Model file for the job. Use its own axes, mm. A direction names the side the tool comes from. Give positions to 0.01 mm unless a question says otherwise; leave off trailing zeros. Write each loop counter-clockwise with the first axis right and the second up, starting at its lowest first coordinate (ties: lowest second). Pieces come first, ordered by that corner, then holes.
```python
from build123d import *

# Parameters (mm, degrees)
SKETCH1_R           = 7.5
SKETCH1_R_2         = 1.7525
BOSS_EXTRUDE1_DEPTH = 6.35


with BuildPart() as part:
    # Sketch1 → Boss-Extrude1 (new body)
    with BuildSketch(Plane.XY):
        with BuildLine():
            Line((100, 110), (80, 110))
            Line((80, 110), (80, 78))
            Line((80, 78), (-3, 78))
            Line((-3, 78), (-3, 110))
            Line((-3, 110), (-27, 110))
            Line((-27, 110), (-27, 78))
            Line((-27, 78), (-110, 78))
            Line((-110, 78), (-110, 110))
            Line((-110, 110), (-130, 110))
            Line((-130, 110), (-130, 63.442887702))
            ThreePointArc((-130, 63.442887702), (-95, 0), (-130, -63.442887702))
            Line((-130, -63.442887702), (-130, -110))
            Line((-130, -110), (-110, -110))
            Line((-110, -110), (-110, -78))
            Line((-110, -78), (-27, -78))
            Line((-27, -78), (-27, -110))
            Line((-27, -110), (-3, -110))
            Line((-3, -110), (-3, -78))
            Line((-3, -78), (80, -78))
            Line((80, -78), (80, -110))
            Line((80, -110), (100, -110))
            Line((100, -110), (100, -63.442887702))
            ThreePointArc((100, -63.442887702), (65, 0), (100, 63.442887702))
            Line((100, 63.442887702), (100, 110))
        make_face()
        with Locations((32.5, 0)):
            Circle(SKETCH1_R, mode=Mode.SUBTRACT)
        with Locations(Location((-67.5, 0, 0), (0, 0, 180))):
            Circle(SKETCH1_R, mode=Mode.SUBTRACT)
        with Locations((-120, 95)):
            Circle(SKETCH1_R_2, mode=Mode.SUBTRACT)
        with Locations(Location((90, 95, 0), (0, 0, 180))):
            Circle(SKETCH1_R_2, mode=Mode.SUBTRACT)
        with Locations((-15, 100)):
            Circle(SKETCH1_R_2, mode=Mode.SUBTRACT)
        with Locations(Location((-15, -100, 0), (0, 0, 180))):
            Circle(SKETCH1_R_2, mode=Mode.SUBTRACT)
        with Locations((90, -95)):
            Circle(SKETCH1_R_2, mode=Mode.SUBTRACT)
        with Locations(Location((-120, -95, 0), (0, 0, 180))):
            Circle(SKETCH1_R_2, mode=Mode.SUBTRACT)
    extrude(amount=BOSS_EXTRUDE1_DEPTH)


solid = part.part
```
1. Probe probe 1 along X at (y, z) = (84.5, 1); probe 2 along X at (y, z) = (95, 4.5); probe 3 along Y at (x, z) = (-15, 2.25). List the from-to ranges inside material, lowest first.
Calculated:
probe 1: x = -130 to -110, -27 to -3, 80 to 100
probe 2: x = -130 to -121.75, -118.25 to -110, -27 to -3, 80 to 88.25, 91.75 to 100
probe 3: y = -110 to -101.75, -98.25 to 98.25, 101.75 to 110
2. Pull direction X, two halves, no side cores. Call faces 1 (the flat face through (-120, -110, 3)), 2 (the flat face through (39, 78, 3)), 3 (the flat face through (-130, -86, 3)): +X half, -X half, draft (parallel to the pull), parting line (faces both ways), or undercut.
Calculated:
face 1: draft
face 2: undercut
face 3: -X half
3. Which spindle directions (+Z, -Z, +X, -X, +Y, -Y) get a long thin tool onto all of the face, cutting with end or side? Do faces 4 (the flat face through (80, 94, 3)), 5 (the flat face through (-69, -78, 3)), 6 (the flat face through (-15, 110, 3)). Say none if no direction does.
Calculated:
face 4: +Z, -Z, +Y
face 5: +Z, -Z, -Y
face 6: +Z, -Z, +X, -X, +Y
4. Pin check, flat tips, straight feed: P1, Ø3, axis at x = 45, z = 3, coming from the +Y side; P2, Ø1.9, axis at x = -59.5, z = 2.5, coming from the -Y side. Stop position of each tip, or through.
Calculated:
P1: stops at y = 78
P2: stops at y = -78
5. Slice it at D-D, the plane y = -48. Write the cut outline in (x, z), and give its area (3 significant figures).
Calculated:
outline: (-112.37, 0) - (82.37, 0) - (82.37, 6.35) - (-112.37, 6.35) - close
area: 1,240 mm2
6. Slice it at A-A, the plane x = 32.5. Write the cut outline in (y, z).
Calculated:
outline: (-78, 0) - (-7.5, 0) - (-7.5, 6.35) - (-78, 6.35) - close; (7.5, 0) - (78, 0) - (78, 6.35) - (7.5, 6.35) - close
7. Slice it at C-C, the plane y = 45. Write the cut outline in (x, z), and give its area (3 significant figures).
Calculated:
outline: (-110, 0) - (80, 0) - (80, 6.35) - (-110, 6.35) - close
area: 1,210 mm2
8. Slice it at B-B, the plane z = 3.5. State how many separate pieces and enclosed holes the cut face has, and give its area (3 significant figures).
Calculated:
separate pieces: 1
enclosed holes: 8
area: 33,300 mm2
